from build123d import *

# Parameters (mm, degrees)
SKETCH_2_R          = 19.5
EXTRUDE_1_DEPTH     = 13
CUT_EXTRUDE_1_DEPTH = 1.5
SKETCH_4_R          = 18.3
CUT_EXTRUDE_2_DEPTH = 11.1
SKETCH_5_R          = 1.05
SKETCH_5_R_2        = 0.6
CUT_EXTRUDE_3_DEPTH = 41.284008974
SKETCH_6_R          = 2.05
CUT_EXTRUDE_4_DEPTH = 1
SKETCH_8_W          = 8.75
SKETCH_8_H          = 7.3
CUT_EXTRUDE_5_DEPTH = 3.25
CUT_EXTRUDE_6_DEPTH = 2


with BuildPart() as part:
    # 草图2 → 凸台-拉伸1 (new body)
    with BuildSketch(Plane.XY):
        with Locations(Location((5.210280057, 9.537965238, 0), (0, 0, 180))):
            Circle(SKETCH_2_R)
    extrude(amount=EXTRUDE_1_DEPTH)

    # 草图3 → 切除-拉伸1 (cut)
    with BuildSketch(Plane.XY):
        with BuildLine():
            ThreePointArc((-2.089466108, -9.474373158), (5.210280057, -10.827576871), (12.510026223, -9.474373158))
            add(Edge.make_bspline(
                [(12.510026223, -9.474373158), (12.542948952, -8.674555972), (12.802081824, -7.965268064), (13.798852187, -6.666991519), (14.542722505, -6.079743438), (15.544339227, -5.564922601)],
                knots=[0, 0, 0, 0, 0.5, 0.5, 1, 1, 1, 1], degree=3))
            ThreePointArc((15.544339227, -5.564922601), (5.210280058, 27.837965238), (-5.123779113, -5.564922601))
            add(Edge.make_bspline(
                [(-5.123779113, -5.564922601), (-4.122162391, -6.079743437), (-3.378292072, -6.666991518), (-2.381521709, -7.965268064), (-2.122388837, -8.674555972), (-2.089466108, -9.474373158)],
                knots=[0, 0, 0, 0, 0.5, 0.5, 1, 1, 1, 1], degree=3))
        make_face()
    extrude(amount=CUT_EXTRUDE_1_DEPTH, mode=Mode.SUBTRACT)

    # 草图4 → 切除-拉伸2 (cut)
    with BuildSketch(Plane.XY):
        with Locations(Location((5.210280057, 9.537965238, 0), (0, 0, 240.328288749))):
            Circle(SKETCH_4_R)
    extrude(amount=CUT_EXTRUDE_2_DEPTH, mode=Mode.SUBTRACT)

    # 草图5 → 切除-拉伸3 (cut, through all)
    with BuildSketch(Plane.XY):
        with Locations(Location((19.360280057, 9.537965238, 0), (0, 0, 180))):
            Circle(SKETCH_5_R)
        with Locations(Location((-8.939719943, 9.537965238, 0), (0, 0, 180))):
            Circle(SKETCH_5_R)
        with Locations((-8.939719943, 15.537965238)):
            Circle(SKETCH_5_R_2)
    extrude(amount=CUT_EXTRUDE_3_DEPTH, mode=Mode.SUBTRACT)

    # 草图6 → 切除-拉伸4 (cut)
    with BuildSketch(Plane.XY.offset(13)):
        with Locations((-8.939719943, 9.537965238)):
            Circle(SKETCH_6_R)
        with Locations((19.360280057, 9.537965238)):
            Circle(SKETCH_6_R)
    extrude(amount=-CUT_EXTRUDE_4_DEPTH, mode=Mode.SUBTRACT)

    # 草图8 → 切除-拉伸5 (cut)
    with BuildSketch(Plane(origin=(0, 0, 3.1), x_dir=(-1, 0, 0), z_dir=(0, 0, -1))):
        with Locations((-5.210300293, -6.312034762)):
            Rectangle(SKETCH_8_W, SKETCH_8_H)
    extrude(amount=-CUT_EXTRUDE_5_DEPTH, mode=Mode.SUBTRACT)

    # 草图9 → 切除-拉伸6 (cut)
    with BuildSketch(Plane(origin=(0, 0, 3.1), x_dir=(-1, 0, 0), z_dir=(0, 0, -1))):
        with BuildLine():
            ThreePointArc((-20.059522462, 24.387207643), (-20.580706206, 23.847053259), (-21.082253473, 23.28861831))
            Line((-21.082253473, 23.28861831), (-18.998862291, 21.205227127))
            Line((-18.998862291, 21.205227127), (-17.938202119, 22.265887299))
            Line((-17.938202119, 22.265887299), (-16.877541947, 23.326547471))
            Line((-16.877541947, 23.326547471), (-18.960933129, 25.409938653))
            ThreePointArc((-18.960933129, 25.409938653), (-19.519368079, 24.908391387), (-20.059522462, 24.387207643))
        make_face()
        with BuildLine():
            Line((8.578302176, 21.205227127), (10.661693358, 23.28861831))
            ThreePointArc((10.661693358, 23.28861831), (10.160146112, 23.847053237), (9.638962389, 24.387207601))
            ThreePointArc((9.638962389, 24.387207601), (9.098807986, 24.908391366), (8.540373014, 25.409938653))
            Line((8.540373014, 25.409938653), (6.456981832, 23.326547471))
            Line((6.456981832, 23.326547471), (7.517642025, 22.265887278))
            Line((7.517642025, 22.265887278), (8.578302176, 21.205227127))
        make_face()
    extrude(amount=-CUT_EXTRUDE_6_DEPTH, mode=Mode.SUBTRACT)


solid = part.part
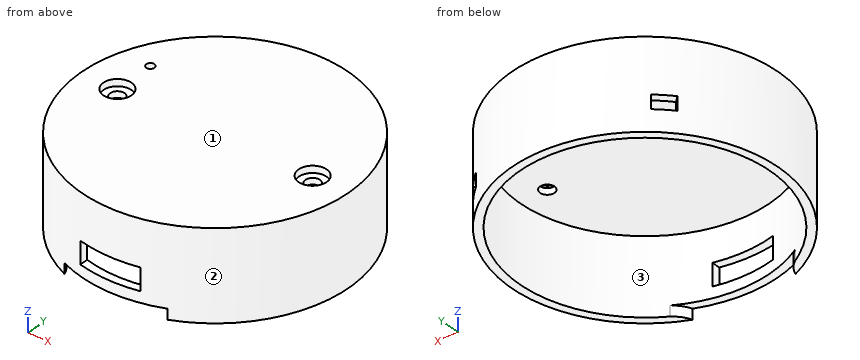
Read the model definition and answer for the solid it produces. Units are mm, in the model's axes. Face numbers are marked on the shaded views. Give positions to 0.01 mm unless a question says otherwise; leave off trailing zeros. Loops run counter-clockwise (first coordinate to the right, second up) from the corner with the lowest first, then second, coordinate; pieces in that order, holes last. Notation, with made-up numbers: M 11,-4 L 64,-4 A34 cw 64,27 Z; hole C -12,50.5 d6. An arc over 180 degrees is marked long. Write each question's results on one line, items separated by ' | '.
1. Section D-D on x = 10.5 is taken. Give the vertices of the cut face in (y, z), plus the area to 3 significant figures.
Values:
outline: M -9.23,1.5 L -7.98,1.5 L -7.98,11.1 L 27.06,11.1 L 27.06,0 L 28.31,0 L 28.31,13 L -9.23,13 Z | area: 97.2 mm^2
2. The mould has two halves that part along Y. Classify the marked faces 1, 2 and 3: pulls with the +Y half, pulls with the -Y half, needs draft (parallel to the pull), parting line crosses it, or undercut.
Values:
face 1: needs draft | face 2: parting line crosses it | face 3: undercut
3. Given pin 1 (5 mm diameter, centred on x = -5, z = 7, fed in from -Y); pin 2 (1.1 mm diameter, centred on x = 6.5, y = -7.5, fed in from -Z); pin 3 (4 mm diameter, centred on y = 20.5, z = 3, fed in from +X); pin 4 (1.9 mm diameter, centred on x = -8.94, y = 9.54, fed in from +Z), each flat-ended and moving along its own axis, determine where each tip first touches the part or whether it passes through.
Values:
pin 1: stops at y = -8.37 | pin 2: stops at z = 11.1 | pin 3: stops at x = 22.53 | pin 4: passes through
4. Section B-B on x = 4.5 is taken. Give the vertices of the cut face in (y, z).
Values:
outline: M -9.95,1.5 L -8.75,1.5 L -8.75,3.1 L -9.95,3.1 Z; M -9.95,6.35 L -8.75,6.35 L -8.75,11.1 L 27.82,11.1 L 27.82,0 L 29.03,0 L 29.03,13 L -9.95,13 Z
5. Section C-C on y = 2.5 is taken. Give the vertices of the cut face in (x, z).
Values:
outline: M -12.98,0 L -11.68,0 L -11.68,11.1 L 22.1,11.1 L 22.1,0 L 23.4,0 L 23.4,13 L -12.98,13 Z
6. Straight lines are drawn through the part: line 1 (Z direction, x = -11, y = 12); line 2 (X direction, y = -2, z = 3.25); line 3 (X direction, y = -3.5, z = 5.75). For each, find the intervals that lie inside material, in ascending order. Write a range as [from, to].
Values:
line 1: z = [11.1, 13] | line 2: x = [-10.51, -8.99], [19.41, 20.93] | line 3: x = [-9.29, -7.63], [18.05, 19.71]
7. Section A-A on z = 4.25 is taken. Give the vertices of the cut face in (x, y), plus the area to 3 significant figures.
Values:
outline: M -9.6,22.23 A19.5 ccw 0.84,-9.46 L 0.84,-8.23 A18.3 cw -8.75,21.37 Z; M -7.48,24.35 L -6.63,23.5 A18.3 cw 17.05,23.5 L 17.9,24.35 A19.5 ccw Z; M 9.59,-9.46 A19.5 ccw 20.02,22.23 L 19.17,21.37 A18.3 cw 9.59,-8.23 Z | area: 125 mm^2
